from build123d import *

# Parameters (mm, degrees)
F0_W     = 20
F0_H     = 32
F1_DEPTH = 2
F2_DEPTH = 4
F0_R     = 3.75
F3_DEPTH = 10


with BuildPart() as f1:
    # F0 (on Top) → F1 (new body)
    with BuildSketch(Plane.XY):
        with BuildLine():
            Line((-12, 2), (-12, 18))
            Line((-12, 18), (-4, 18))
            Line((-4, 18), (-26, 34.130678))
            ThreePointArc((-26, 34.130678), (-24.705545, 32.243045), (-24.25, 30))
            ThreePointArc((-24.25, 30), (-27.107282, 25.030626), (-32.839454, 25))
            Line((-32.839454, 25), (-12, 2))
        make_face()
        with BuildLine():
            Line((26, 34.130678), (4, 18))
            Line((4, 18), (12, 18))
            Line((12, 18), (12, 2))
            Line((12, 2), (32.839454, 25))
            ThreePointArc((32.839454, 25), (25.397931, 26.55276), (26, 34.130678))
        make_face()
        with BuildLine():
            Line((32.839454, -25), (12, -2))
            Line((12, -2), (12, -18))
            Line((12, -18), (4, -18))
            Line((4, -18), (26, -34.130678))
            ThreePointArc((26, -34.130678), (25.397931, -26.55276), (32.839454, -25))
        make_face()
        with BuildLine():
            Line((-12, -18), (-12, -2))
            Line((-12, -2), (-32.839454, -25))
            ThreePointArc((-32.839454, -25), (-27.107282, -25.030626), (-24.25, -30))
            ThreePointArc((-24.25, -30), (-24.705545, -32.243045), (-26, -34.130678))
            Line((-26, -34.130678), (-4, -18))
            Line((-4, -18), (-12, -18))
        make_face()
        Polygon((-4, 18), (-12, 18), (-12, 2), (-12, -2), (-12, -18), (-4, -18), (4, -18), (12, -18), (12, -2), (12, 2), (12, 18), (4, 18), align=None)
        Rectangle(F0_W, F0_H, mode=Mode.SUBTRACT)
        Rectangle(F0_W, F0_H)
    extrude(amount=F1_DEPTH)

    # F0 (on Top) → F2 (join)
    with BuildSketch(Plane.XY):
        Polygon((-4, 18), (-12, 18), (-12, 2), (-12, -2), (-12, -18), (-4, -18), (4, -18), (12, -18), (12, -2), (12, 2), (12, 18), (4, 18), align=None)
        Rectangle(F0_W, F0_H, mode=Mode.SUBTRACT)
    extrude(amount=F2_DEPTH)

    # F0 (on Top) → F3 (join)
    with BuildSketch(Plane.XY):
        with BuildLine():
            ThreePointArc((-24.25, -30), (-27.107282, -25.030626), (-32.839454, -25))
            ThreePointArc((-32.839454, -25), (-34.602069, -33.44724), (-26, -34.130678))
            ThreePointArc((-26, -34.130678), (-24.705545, -32.243045), (-24.25, -30))
        make_face()
        with Locations((-30, -30)):
            Circle(F0_R, mode=Mode.SUBTRACT)
        with BuildLine():
            ThreePointArc((35.75, -30), (34.969374, -27.107282), (32.839454, -25))
            ThreePointArc((32.839454, -25), (25.397931, -26.55276), (26, -34.130678))
            ThreePointArc((26, -34.130678), (32.243045, -35.294455), (35.75, -30))
        make_face()
        with Locations((30, -30)):
            Circle(F0_R, mode=Mode.SUBTRACT)
        with BuildLine():
            ThreePointArc((35.75, 30), (32.243045, 35.294455), (26, 34.130678))
            ThreePointArc((26, 34.130678), (25.397931, 26.55276), (32.839454, 25))
            ThreePointArc((32.839454, 25), (34.969374, 27.107282), (35.75, 30))
        make_face()
        with Locations((30, 30)):
            Circle(F0_R, mode=Mode.SUBTRACT)
        with BuildLine():
            ThreePointArc((-24.25, 30), (-24.705545, 32.243045), (-26, 34.130678))
            ThreePointArc((-26, 34.130678), (-34.602069, 33.44724), (-32.839454, 25))
            ThreePointArc((-32.839454, 25), (-27.107282, 25.030626), (-24.25, 30))
        make_face()
        with Locations((-30, 30)):
            Circle(F0_R, mode=Mode.SUBTRACT)
    extrude(amount=F3_DEPTH)


solid = f1.part
Work out the finished part from the listing and answer in its coordinate system (mm). A direction names the side the tool comes from. Round coordinates to 2 decimals unless told otherwise and drop trailing zeros. Write each loop counter-clockwise with the first axis right and the second up, starting at its lowest first coordinate (ties: lowest second). Pieces come first, ordered by that corner, then holes. Notation, with made-up numbers: (17.25, -33) - (69.25, -33) arc R23 cw to (69.25, -2) - close; hole circle Ø6 at (51.5, -21). An arc over 180 degrees is marked (long way). Answer in a Markdown table with one row per item. Add a question column.
1. The mould has two halves that part along Y. Classify faces 4 (the flat face through (-1, 1, 0)), 5 (the flat face through (0, 18, 2)), 6 (the flat face through (-10, 0, 3)): +Y half, -Y half, draft (parallel to the pull), parting line (faces both ways), or undercut.
2. A cutting plane is placed at D-D, the plane x = -30. Determine the outline of the cut face in (y, z), and give its area (3 significant figures).
3. Find the intervals of material crossed by line 1 along Y through (x, z) = (30, 3.5); line 2 along Y through (x, z) = (0, 3.25); line 3 along Z through (x, y) = (-26.5, 18.5), in increasing order. Write a range as from..to.
4. A cutting plane is placed at C-C, the plane y = 20.5. Determine the outline of the cut face in (x, z).
5. For faces 1 (the flat face through (15.154, 26.178, 0.986)), 2 (the flat face through (12, 0, 3)), 3 (the flat face through (-22.6, 13.7, 1)), determine the directions among +Z, -Z, +X, -X, +Y, -Y from which every point of the face is accessible in a straight line to the end or side of a thin tool.
6. A cutting plane is placed at B-B, the plane y = -0.5. Determine the outline of the cut face in (x, z).
7. Given pin 1 (12 mm diameter, centred on x = -6, y = -5, fed in from +Z); pin 2 (0.6 mm diameter, centred on x = 2, z = 3, fed in from -Y); pin 3 (5 mm diameter, centred on y = -15.5, z = 5.5, fed in from +X), each flat-ended and moving along its own axis, determine where each tip first touches the part or whether it passes through.
8. A cutting plane is placed at A-A, the plane z = 6. Determine the outline of the cut face in (x, y).
Worked out:
| question | item | result |
|---|---|---|
| 1 | face 4 | draft |
| 1 | face 5 | +Y half |
| 1 | face 6 | undercut |
| 2 | outline | (-35.75, 0) - (-33.75, 0) - (-33.75, 10) - (-35.75, 10) - close; (-26.25, 0) - (-21.87, 0) - (-21.87, 2) - (-24.25, 2) - (-24.25, 10) - (-26.25, 10) - close; (21.87, 0) - (26.25, 0) - (26.25, 10) - (24.25, 10) - (24.25, 2) - (21.87, 2) - close; (33.75, 0) - (35.75, 0) - (35.75, 10) - (33.75, 10) - close |
| 2 | area | 89.5 mm^2 |
| 3 | line 1 | -35.75..-33.75, -26.25..-24.25, 24.25..26.25, 33.75..35.75 |
| 3 | line 2 | -18..-16, 16..18 |
| 3 | line 3 | 0..2 |
| 4 | outline | (-28.76, 0) - (-7.41, 0) - (-7.41, 2) - (-28.76, 2) - close; (7.41, 0) - (28.76, 0) - (28.76, 2) - (7.41, 2) - close |
| 5 | face 1 | +Z, -Z, +Y |
| 5 | face 2 | +Z, +X |
| 5 | face 3 | +Z, -Z, -X |
| 6 | outline | (-12, 0) - (12, 0) - (12, 4) - (10, 4) - (10, 2) - (-10, 2) - (-10, 4) - (-12, 4) - close |
| 7 | pin 1 | z = 4 |
| 7 | pin 2 | y = -18 |
| 7 | pin 3 | x = 12 |
| 8 | outline | (-26, -34.13) arc R5.75 ccw to (-24.25, -30) arc R5.75 ccw (long way) to start; (-26, 34.13) arc R5.75 ccw (long way) to (-24.25, 30) arc R5.75 ccw to start; (32.84, -25) arc R5.75 ccw (long way) to (35.75, -30) arc R5.75 ccw to start; (32.84, 25) arc R5.75 ccw to (35.75, 30) arc R5.75 ccw (long way) to start; hole circle Ø7.5 at (-30, -30); hole circle Ø7.5 at (-30, 30); hole circle Ø7.5 at (30, -30); hole circle Ø7.5 at (30, 30) |
